Geometry: final body of the model. Coordinates: model frame, mm. Give positions to 0.01 mm unless a question says otherwise; leave off trailing zeros. Write each loop counter-clockwise with the first axis right and the second up, starting at its lowest first coordinate (ties: lowest second). Pieces come first, ordered by that corner, then holes.
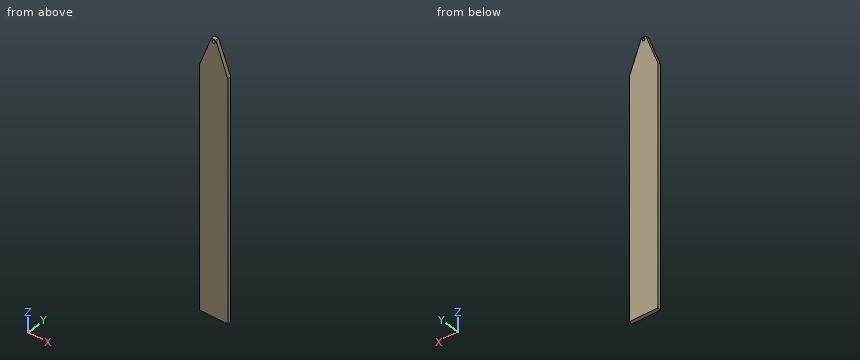
from build123d import *

# Parameters (mm, degrees)
F0_W     = 31.75
F0_H     = 3.9878
F1_DEPTH = 152.4
F2_R     = 1.5875
F3_DEPTH = 3.9888


with BuildPart() as f1:
    # F0 (on Top) → F1 (new body, symmetric)
    with BuildSketch(Plane.XY):
        Rectangle(F0_W, F0_H)
    extrude(amount=F1_DEPTH, both=True)

    # F2 (on face) → F3 (cut, through all)
    with BuildSketch(Plane.XZ.offset(1.9939)):
        with Locations((0, 149.86)):
            Circle(F2_R)
        Polygon((-15.875, 116.70918), (-2.472009, 152.4), (-15.875, 152.4), align=None)
        Polygon((15.875, 152.4), (2.472009, 152.4), (15.875, 116.70918), align=None)
    extrude(amount=-F3_DEPTH, mode=Mode.SUBTRACT)


solid = f1.part
Q1. Section A-A on y = 1.15. Output: boundary loops of the cut face in (x, z) (1 decimal).
Filled sheet:
outline: (-15.9, -152.4) - (15.9, -152.4) - (15.9, 116.7) - (2.5, 152.4) - (-2.5, 152.4) - (-15.9, 116.7) - close; hole circle Ø3.2 at (0, 149.9)
Q2. Section B-B on x = 9.5. Output: boundary loops of the cut face in (y, z), plus the area to 3 significant figures.
Filled sheet:
outline: (-1.99, -152.4) - (1.99, -152.4) - (1.99, 133.69) - (-1.99, 133.69) - close
area: 1,140 mm2
Q3. Pin query (flat end, axial travel): P1, Ø1.9, axis at x = 0, z = 149.86, coming from the +Y side. Return the tip coordinate at first contact, or that it passes through.
Filled sheet:
P1: passes through
Q4. Ray query, line 1 along Z through (x, y) = (0, -0.4); line 2 along X through (y, z) = (-0.3, 149.86); line 3 along X through (y, z) = (-0.65, 134). Return the intervals inside material, ascending.
Filled sheet:
line 1: z = -152.4 to 148.27, 151.45 to 152.4
line 2: x = -3.43 to -1.59, 1.59 to 3.43
line 3: x = -9.38 to 9.38
